```python
from build123d import *

# Parameters (mm, degrees)
SKETCH1_W           = 15
SKETCH1_H           = 7
BOSS_EXTRUDE1_DEPTH = 0.75
BOSS_EXTRUDE2_DEPTH = 1.5


with BuildPart() as part:
    # Sketch1 → Boss-Extrude1 (new body)
    with BuildSketch(Plane(origin=(0, 0, 0), x_dir=(1, 0, 0), z_dir=(0, 1, 0))):
        Rectangle(SKETCH1_W, SKETCH1_H)
    extrude(amount=BOSS_EXTRUDE1_DEPTH)

    # Sketch2 → Boss-Extrude2 (add)
    with BuildSketch(Plane(origin=(0, 0.75, 0), x_dir=(1, 0, 0), z_dir=(0, 1, 0))):
        Polygon((6.962231563, -2.748114094), (6.353774698, 2.543552573), (6.161909381, 2.543552573), (4.35031917, -1.798327769), (2.547209194, 2.543552573), (2.348983699, 2.543552573), (1.738406776, -2.748114094), (2.214359968, -2.748114094), (2.654272161, 1.051031205), (4.231595879, -2.748114094), (4.460562225, -2.748114094), (6.046366178, 1.051031205), (6.483098283, -2.748114094), align=None)
        Polygon((-1.043110318, 2.543552573), (-3.010524848, -2.748114094), (-2.495350569, -2.748114094), (-1.866753146, -1.052067085), (-0.024422083, -1.052067085), (0.67095719, -2.748114094), (1.195671734, -2.748114094), (-0.975268437, 2.543552573), align=None)
        Polygon((-0.990108849, 1.302258169), (-0.247028253, -0.509332042), (-1.664287535, -0.509332042), align=None, mode=Mode.SUBTRACT)
        Polygon((-3.55325989, 2.543552573), (-4.107655256, 2.543552573), (-5.283227839, 0.35883202), (-6.457740392, 2.543552573), (-7.013195788, 2.543552573), (-5.52067442, -0.232664374), (-5.52067442, -2.748114094), (-5.045781258, -2.748114094), (-5.045781258, -0.232664374), align=None)
    extrude(amount=BOSS_EXTRUDE2_DEPTH)


solid = part.part
```
Can you work these out from the model? Positions are in its coordinate system, mm. A direction names the side the tool comes from. Coordinates: 2 decimals unless noted, no trailing zeros. Loops run counter-clockwise (first coordinate to the right, second up) from the corner with the lowest first, then second, coordinate; pieces in that order, holes last.
1) Imagine slicing it at B-B on z = 2.5. List the corners of the cut face in (x, y) for me.
2) Imagine slicing it at C-C on x = -1.5. List the corners of the cut face in (y, z) for me.
3) Which directions (+Z, -Z, +X, -X, +Y, -Y) give clear straight access to the entire face, cutting with the end or side of a thin tool? Please do faces 4 (the flat face through (-1, 1, 0.509)), 5 (the flat face through (-5.862, 1.49, -1.436)), 6 (the flat face through (-1, 1, 1.052)).
4) I need wall thicknesses on probe 1 along X at (y, z) = (1.35, 2.5); probe 2 along X at (y, z) = (1.5, 2.25); probe 3 along X at (y, z) = (2.2, -1.5). Which ranges of each line are inside material? Lowest first, please.
5) Thinking about a two-plate mould opening in Z: for faces 1 (the flat face through (-4.687, 1.49, -1.466)), 2 (the flat face through (-5.521, 1, 1)), 3 (the flat face through (-0.624, 1.49, -0.409)), which applies, pulls with the +Z half, pulls with the -Z half, needs draft (parallel to the pull), parting line crosses it, or undercut?
6) Imagine slicing it at A-A on y = 1.05. State how many separate pieces and enclosed holes the cut face has, plus the area to 3 significant figures.
7) Imagine slicing it at D-D on x = -4.25. List the corners of the cut face in (y, z) for me, plus the area to 3 significant figures.
8) For pin 1 (0.5 mm diameter, centred on x = 7, y = 1.5, fed in from +Z); pin 2 (0.6 mm diameter, centred on x = -4, y = 1.5, fed in from -Z); pin 3 (0.8 mm diameter, centred on y = 1.5, z = 1, fed in from +X), each with a flat end and sliding along its axis, tell me the tip position at first contact or that it passes through.
Completed:
1. outline: (-7.5, 0) - (7.5, 0) - (7.5, 0.75) - (6.93, 0.75) - (6.93, 2.25) - (6.45, 2.25) - (6.45, 0.75) - (4.56, 0.75) - (4.56, 2.25) - (4.13, 2.25) - (4.13, 0.75) - (2.24, 0.75) - (2.24, 2.25) - (1.77, 2.25) - (1.77, 0.75) - (1.09, 0.75) - (1.09, 2.25) - (0.57, 2.25) - (0.57, 0.75) - (-2.4, 0.75) - (-2.4, 2.25) - (-2.92, 2.25) - (-2.92, 0.75) - (-5.05, 0.75) - (-5.05, 2.25) - (-5.52, 2.25) - (-5.52, 0.75) - (-7.5, 0.75) - close
2. outline: (0, -3.5) - (0.75, -3.5) - (0.75, -1.31) - (2.25, -1.31) - (2.25, 0.07) - (0.75, 0.07) - (0.75, 0.51) - (2.25, 0.51) - (2.25, 1.05) - (0.75, 1.05) - (0.75, 3.5) - (0, 3.5) - close
3. face 4: +Y
3. face 5: -Z, +Y
3. face 6: +Z, +Y
4. probe 1: x = -5.52 to -5.05, -2.92 to -2.4, 0.57 to 1.09, 1.77 to 2.24, 4.13 to 4.56, 6.45 to 6.93
4. probe 2: x = -5.52 to -5.05, -2.83 to -2.31, 0.47 to 0.99, 1.8 to 2.27, 4.02 to 4.67, 6.43 to 6.9
4. probe 3: x = -6.45 to -5.9, -4.67 to -4.11, -1.43 to -0.55, 2.23 to 2.98, 5.73 to 6.47
5. face 1: pulls with the -Z half
5. face 2: needs draft
5. face 3: undercut
6. separate pieces: 3
6. enclosed holes: 1
6. area: 18.8 mm2
7. outline: (0, -3.5) - (0.75, -3.5) - (0.75, -2.28) - (2.25, -2.28) - (2.25, -1.25) - (0.75, -1.25) - (0.75, 3.5) - (0, 3.5) - close
7. area: 6.80 mm2
8. pin 1: stops at z = 2.75
8. pin 2: stops at z = -2.54
8. pin 3: stops at x = 6.81
